Build history of the part. All positions in model axes, mm. A direction names the side the tool comes from. Give positions to 0.01 mm unless a question says otherwise; leave off trailing zeros. Write each loop counter-clockwise with the first axis right and the second up, starting at its lowest first coordinate (ties: lowest second). Pieces come first, ordered by that corner, then holes. Notation, with made-up numbers: (61, 45.5) -> (100, 45.5) arc R24 cw to (100, 75.5) -> close; hole circle Ø5 at (73, -3). An arc over 180 degrees is marked (long way). Put each result on its own line as item: value.
from build123d import *

# Parameters (mm, degrees)
F0_W      = 200
F0_H      = 337
F1_DEPTH  = 18.1
F2_W      = 25
F2_H      = 18.6
F2_W_2    = 150
F3_DEPTH  = 10
F5_DEPTH  = 25
F6_W      = 7
F6_H      = 209.4
F7_DEPTH  = 10
F8_W      = 7
F8_H      = 109
F9_DEPTH  = 10
F10_W     = 5
F10_H     = 18.6
F11_DEPTH = 13


with BuildPart() as f1:
    # F0 (on Top) → F1 (new body)
    with BuildSketch(Plane.XY):
        Rectangle(F0_W, F0_H)
    extrude(amount=F1_DEPTH)

    # F2 (on face) → F3 (cut)
    with BuildSketch(Plane.XY.offset(18.1)):
        with Locations((-87.5, -50.2)):
            Rectangle(F2_W, F2_H)
        with Locations((-62.5, -50.2)):
            Rectangle(F2_W, F2_H)
        with Locations((25, -50.2)):
            Rectangle(F2_W_2, F2_H)
        with Locations((112.5, -50.2)):
            Rectangle(F2_W, F2_H)
        with Locations((137.5, -50.2)):
            Rectangle(F2_W, F2_H)
    extrude(amount=-F3_DEPTH, mode=Mode.SUBTRACT)

    # F4 (on face) → F5 (cut)
    with BuildSketch(Plane.XY.offset(8.1)):
        with BuildLine():
            Line((-52.5, -50.2), (-50, -50.2))
            Line((-50, -50.2), (-47.5, -50.2))
            ThreePointArc((-47.5, -50.2), (-50, -47.7), (-52.5, -50.2))
        make_face()
        with BuildLine():
            Line((-47.5, -50.2), (-50, -50.2))
            Line((-50, -50.2), (-52.5, -50.2))
            ThreePointArc((-52.5, -50.2), (-50, -52.7), (-47.5, -50.2))
        make_face()
        with BuildLine():
            ThreePointArc((52.5, -50.2), (50, -47.7), (47.5, -50.2))
            Line((47.5, -50.2), (50, -50.2))
            Line((50, -50.2), (52.5, -50.2))
        make_face()
        with BuildLine():
            Line((50, -50.2), (47.5, -50.2))
            ThreePointArc((47.5, -50.2), (50, -52.7), (52.5, -50.2))
            Line((52.5, -50.2), (50, -50.2))
        make_face()
    extrude(amount=-F5_DEPTH, mode=Mode.SUBTRACT)

    # F6 (on face) → F7 (cut)
    with BuildSketch(Plane.XY.offset(18.1)):
        with Locations((-91.5, 63.8)):
            Rectangle(F6_W, F6_H)
    extrude(amount=-F7_DEPTH, mode=Mode.SUBTRACT)

    # F8 (on face) → F9 (cut)
    with BuildSketch(Plane.XY.offset(18.1)):
        with Locations((-91.5, -114)):
            Rectangle(F8_W, F8_H)
    extrude(amount=-F9_DEPTH, mode=Mode.SUBTRACT)

    # F10 (on face) → F11 (join)
    with BuildSketch(Plane.XY.offset(18.1)):
        with Locations((-97.5, -50.2)):
            Rectangle(F10_W, F10_H)
    extrude(amount=-F11_DEPTH)


solid = f1.part
1) Slice it at C-C (y = -19.5). Write the cut outline in (x, z).
Filled sheet:
outline: (-100, 0) -> (100, 0) -> (100, 18.1) -> (-88, 18.1) -> (-88, 8.1) -> (-95, 8.1) -> (-95, 18.1) -> (-100, 18.1) -> close
2) Tool access for faces 1 (the flat face through (5, -59.5, 13)), 2 (the flat face through (-100, -2, 9)), 3 (the flat face through (-95, -2, 13)): list every direction of +Z, -Z, +X, -X, +Y, -Y with a clear straight run to the whole face (end or side of a thin tool).
Filled sheet:
face 1: +Z, +X
face 2: +Z, -Z, -X, +Y, -Y
face 3: +Z, +Y, -Y
3) Slice it at B-B (x = 27). Write the cut outline in (y, z), plus the area to 3 significant figures.
Filled sheet:
outline: (-168.5, 0) -> (168.5, 0) -> (168.5, 18.1) -> (-40.9, 18.1) -> (-40.9, 8.1) -> (-59.5, 8.1) -> (-59.5, 18.1) -> (-168.5, 18.1) -> close
area: 5,910 mm2
4) Slice it at A-A (z = 12). Write the cut outline in (x, y), plus the area to 3 significant figures.
Filled sheet:
outline: (-100, -168.5) -> (-95, -168.5) -> (-95, 168.5) -> (-100, 168.5) -> close; (-88, -168.5) -> (100, -168.5) -> (100, -59.5) -> (-88, -59.5) -> close; (-88, -40.9) -> (100, -40.9) -> (100, 168.5) -> (-88, 168.5) -> close
area: 61,500 mm2
5) Wall check: L1, parallel to X at y = -50.2, z = 4.5; L2, parallel to Y at x = -50, z = 6.5; L3, parallel to X at y = 82.5, z = 15.5. Give the ranges that are in metal, low to high.
Filled sheet:
L1: -100 to -52.5, -47.5 to 47.5, 52.5 to 100
L2: -168.5 to -52.7, -47.7 to 168.5
L3: -100 to -95, -88 to 100
6) Pull direction X, two halves, no side cores. Call faces 4 (the flat face through (100, -2, 9)), 5 (the flat face through (-1, 2, 0)), 6 (the flat face through (-88, -115, 13)): released by +X, released by -X, zero draft, split by the parting line, or undercut.
Filled sheet:
face 4: released by +X
face 5: zero draft
face 6: undercut
